```python
from build123d import *

# Parameters (mm, degrees)
SKETCH1_R           = 2.5
BOSS_EXTRUDE1_DEPTH = 3.5
BOSS_EXTRUDE2_START = 3.5
SKETCH1_3_R         = 2.5
BOSS_EXTRUDE2_DEPTH = 35
CHAMFER1_SIZE       = 0.5


with BuildPart() as part:
    # Sketch1 → Boss-Extrude1 (new body)
    with BuildSketch(Plane(origin=(0, 0, 0), x_dir=(1, 0, 0), z_dir=(0, 1, 0))):
        Polygon((-5.080682369, 0), (-2.540341184, -4.4), (2.540341184, -4.4), (5.080682369, 0), (2.540341184, 4.4), (-2.540341184, 4.4), align=None)
        Circle(SKETCH1_R, mode=Mode.SUBTRACT)
        Circle(SKETCH1_R)
    extrude(amount=BOSS_EXTRUDE1_DEPTH)

    # Sketch1<3> → Boss-Extrude2 (add)
    with BuildSketch(Plane(origin=(0, 0, 0), x_dir=(1, 0, 0), z_dir=(0, 1, 0)).offset(BOSS_EXTRUDE2_START)):
        with Locations(Location((0, 0, 0), (0, 0, 270))):
            Circle(SKETCH1_3_R)
    extrude(amount=BOSS_EXTRUDE2_DEPTH)

    # Chamfer1
    chamfer1_edges = [part.edges().sort_by_distance(p)[0] for p in [
        (0, 38.5, -2.5),
    ]]
    chamfer(chamfer1_edges, length=CHAMFER1_SIZE)


solid = part.part
```
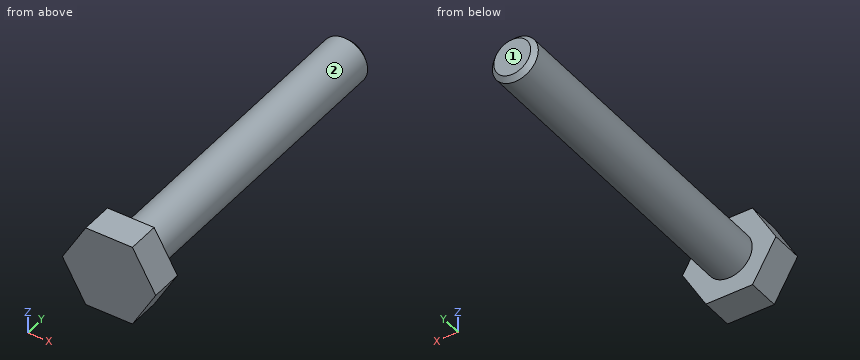
Read the model definition and answer for the solid it produces. Units are mm, in the model's axes. Face numbers are marked on the shaded views. A direction names the side the tool comes from. Give positions to 0.01 mm unless a question says otherwise; leave off trailing zeros. Write each loop counter-clockwise with the first axis right and the second up, starting at its lowest first coordinate (ties: lowest second). Pieces come first, ordered by that corner, then holes. Notation, with made-up numbers: (11.5, 2.5) -> (40.5, 2.5) arc R27 cw to (40.5, 36.5) -> close; hole circle Ø9 at (75, 42.25). An arc over 180 degrees is marked (long way). Answer as a JSON object with one key per item and string values.
1) Straight lines are drawn through the part: probe 1 along Y at (x, z) = (1, -3.5); probe 2 along Z at (x, y) = (-1.5, 10). For each, find the intervals that lie inside material, in ascending order. Write a range as from..to.
Findings below:
{"probe 1": "y = 0..3.5", "probe 2": "z = -2..2"}
2) Section D-D on x = -3.25 is taken. Write down the section's boundary in (y, z), then the cut area to 3 significant figures.
Findings below:
{"outline": "(0, -3.17) -> (3.5, -3.17) -> (3.5, 3.17) -> (0, 3.17) -> close", "area": "22.2 mm^2"}
3) Section B-B on y = 11 is taken. Write down the section's boundary in (x, z), then the cut area to 3 significant figures.
Findings below:
{"outline": "circle Ø5 at (0, 0)", "area": "19.6 mm^2"}
4) Flat-ended cylindrical pins translate along their axes: pin 1 Ø1 at (y, z) = (9, 1.5) entering from -X; pin 2 Ø3 at (y, z) = (8.5, -2) entering from -X; pin 3 Ø3 at (y, z) = (13.5, 2.5) entering from +X. Find the tip coordinate at first contact, or state that the pin passes through.
Findings below:
{"pin 1": "stops at x = -2.29", "pin 2": "stops at x = -2.45", "pin 3": "stops at x = 2.29"}
5) Section A-A on x = 0 is taken. Write down the section's boundary in (y, z).
Findings below:
{"outline": "(0, -4.4) -> (3.5, -4.4) -> (3.5, -2.5) -> (38, -2.5) -> (38.5, -2) -> (38.5, 2) -> (38, 2.5) -> (3.5, 2.5) -> (3.5, 4.4) -> (0, 4.4) -> close"}
6) A tool of negligible diameter and unlimited length cuts with its end or side. For the marked faces 1 and 2, from which of +Z, -Z, +X, -X, +Y, -Y can it reach the whole face along a straight path? Write none if from no direction.
Findings below:
{"face 1": "+Z, -Z, +X, -X, +Y", "face 2": "+Y"}
7) Section C-C on z = 3 is taken. Write down the section's boundary in (x, y), then the cut area to 3 significant figures.
Findings below:
{"outline": "(-3.35, 0) -> (3.35, 0) -> (3.35, 3.5) -> (-3.35, 3.5) -> close", "area": "23.4 mm^2"}
